```python
from build123d import *

# Parameters (mm, degrees)
SKETCH1_R           = 0.2415
BOSS_EXTRUDE1_DEPTH = 0.34
SKETCH2_R           = 2.75
BOSS_EXTRUDE2_DEPTH = 0.2
SKETCH3_R           = 2.55
BOSS_EXTRUDE3_DEPTH = 2.13
FILLET1_R           = 0.2
FILLET2_R           = 0.5
SKETCH4_R           = 0.241
BOSS_EXTRUDE4_DEPTH = 6


with BuildPart() as part:
    # Sketch1 → Boss-Extrude1 (new body)
    with BuildSketch(Plane.XY):
        with BuildLine():
            Line((99.541959491, 58.334320384), (100.320738424, 57.55554145))
            ThreePointArc((100.320738424, 57.55554145), (100.391449102, 57.526252128), (100.462159781, 57.55554145))
            Line((100.462159781, 57.55554145), (101.146639145, 58.240020814))
            ThreePointArc((101.146639145, 58.240020814), (101.175928467, 58.310731493), (101.146639145, 58.381442171))
            Line((101.146639145, 58.381442171), (100.367860211, 59.160221104))
            ThreePointArc((100.367860211, 59.160221104), (100.339288016, 59.218977235), (100.353096237, 59.282836347))
            ThreePointArc((100.353096237, 59.282836347), (96.008801273, 62.693379322), (99.419344248, 58.349084358))
            ThreePointArc((99.419344248, 58.349084358), (99.48320336, 58.362892578), (99.541959491, 58.334320384))
        make_face()
        with Locations((97.975618784, 61.99656181)):
            Circle(SKETCH1_R, mode=Mode.SUBTRACT)
        with Locations((99.245618784, 60.72656181)):
            Circle(SKETCH1_R, mode=Mode.SUBTRACT)
        with Locations((96.705618784, 60.72656181)):
            Circle(SKETCH1_R, mode=Mode.SUBTRACT)
    extrude(amount=BOSS_EXTRUDE1_DEPTH)

    # Sketch2 → Boss-Extrude2 (add)
    with BuildSketch(Plane.XY.offset(0.34)):
        with Locations((97.975618784, 60.72656181)):
            Circle(SKETCH2_R)
    extrude(amount=BOSS_EXTRUDE2_DEPTH)

    # Sketch3 → Boss-Extrude3 (add)
    with BuildSketch(Plane.XY.offset(0.54)):
        with Locations((97.975618784, 60.72656181)):
            Circle(SKETCH3_R)
    extrude(amount=BOSS_EXTRUDE3_DEPTH)

    # Fillet1
    fillet1_edges = [part.edges().sort_by_distance(p)[0] for p in [
        (95.425618784, 60.72656181, 0.54),
    ]]
    fillet(fillet1_edges, radius=FILLET1_R - 0.0001)  # a hair under: the kernel refuses the full size

    # Fillet2
    fillet2_edges = [part.edges().sort_by_distance(p)[0] for p in [
        (95.425618784, 60.72656181, 2.67),
    ]]
    fillet(fillet2_edges, radius=FILLET2_R)

    # Sketch4 → Boss-Extrude4 (add)
    with BuildSketch(Plane(origin=(0, 0, 0.34), x_dir=(-1, 0, 0), z_dir=(0, 0, -1))):
        with Locations(Location((-99.245618784, 60.72656181, 0), (0, 0, 180))):
            Circle(SKETCH4_R)
        with Locations(Location((-97.975618784, 61.99656181, 0), (0, 0, 180))):
            Circle(SKETCH4_R)
        with Locations(Location((-96.705618784, 60.72656181, 0), (0, 0, 180))):
            Circle(SKETCH4_R)
    extrude(amount=BOSS_EXTRUDE4_DEPTH)


solid = part.part
```
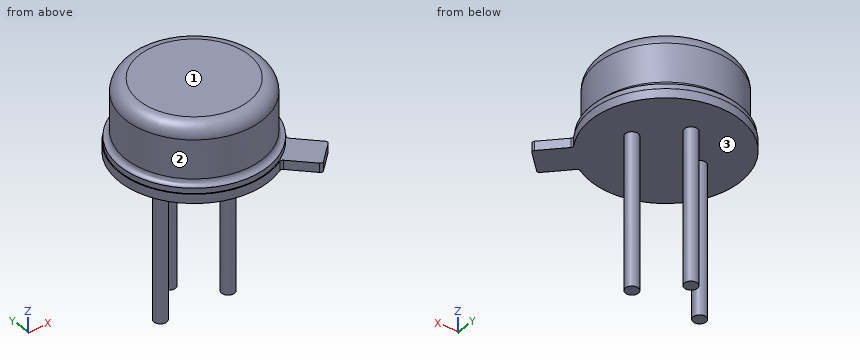
Read the model definition and answer for the solid it produces. Units are mm, in the model's axes. Face numbers are marked on the shaded views. Give positions to 0.01 mm unless a question says otherwise; leave off trailing zeros. Write each loop counter-clockwise with the first axis right and the second up, starting at its lowest first coordinate (ties: lowest second). Pieces come first, ordered by that corner, then holes. Notation, with made-up numbers: (43, 4) - (80, 4) arc R20 cw to (80, 9) - close; hole circle Ø7 at (57.25, -3.5). An arc over 180 degrees is marked (long way). Write item = value, one per line. Start each with the question number.
Item 1: Each of these flat-tipped pins is pushed along its axis until it touches: P1, Ø3, axis at y = 58, z = 0.5, coming from the -X side; P2, Ø2, axis at x = 99.5, z = 1.5, coming from the -Y side. Where does it stop, or does it pass through?
Item 2: Find section B-B (z = 1.25). Give the vertices of the cut face in (x, y).
Item 3: Find section A-A (z = -2). Give the vertices of the cut face in (x, y), then the cut area to 3 significant figures.
Item 4: The mould has two halves that part along Z. Classify the marked faces 1, 2 and 3: +Z half, -Z half, draft (parallel to the pull), parting line (faces both ways), or undercut.
Item 5: Find the intervals of material crossed by probe 1 along Z at (x, y) = (96.1, 61.15); probe 2 along Y at (x, z) = (98, -1.25); probe 3 along Z at (x, y) = (100.7, 58.45), in increasing order. Write a range as [from, to].
Response:
q1.P1 = 95.48
q1.P2 = 58.23
q2.outline = circle Ø5.1 at (97.98, 60.73)
q3.outline = circle Ø0.48 at (96.71, 60.73); circle Ø0.48 at (97.98, 62); circle Ø0.48 at (99.25, 60.73)
q3.area = 0.547 mm²
q4.face_1 = +Z half
q4.face_2 = draft
q4.face_3 = -Z half
q5.probe_1 = [0, 2.67]
q5.probe_2 = [61.76, 62.24]
q5.probe_3 = [0, 0.34]
